The figure shows three views and two pictorial views of one solid part (mm, origin at its lowest corner). Answer the questions. Round coordinates to 2 decimals unless told otherwise and drop trailing zeros. Order: outer loops, then holes, each group sorted by start corner. A loop starts at its lowest first (then second) coordinate and runs counter-clockwise, first axis right, second up. Notation, with made-up numbers: (31, 88) - (77, 88) arc R13 ccw to (77, 94) - close; hole circle Ø7 at (-37.75, -13.75). An arc over 180 degrees is marked (long way). Use CSV: the item, a comma, the result in double quotes.
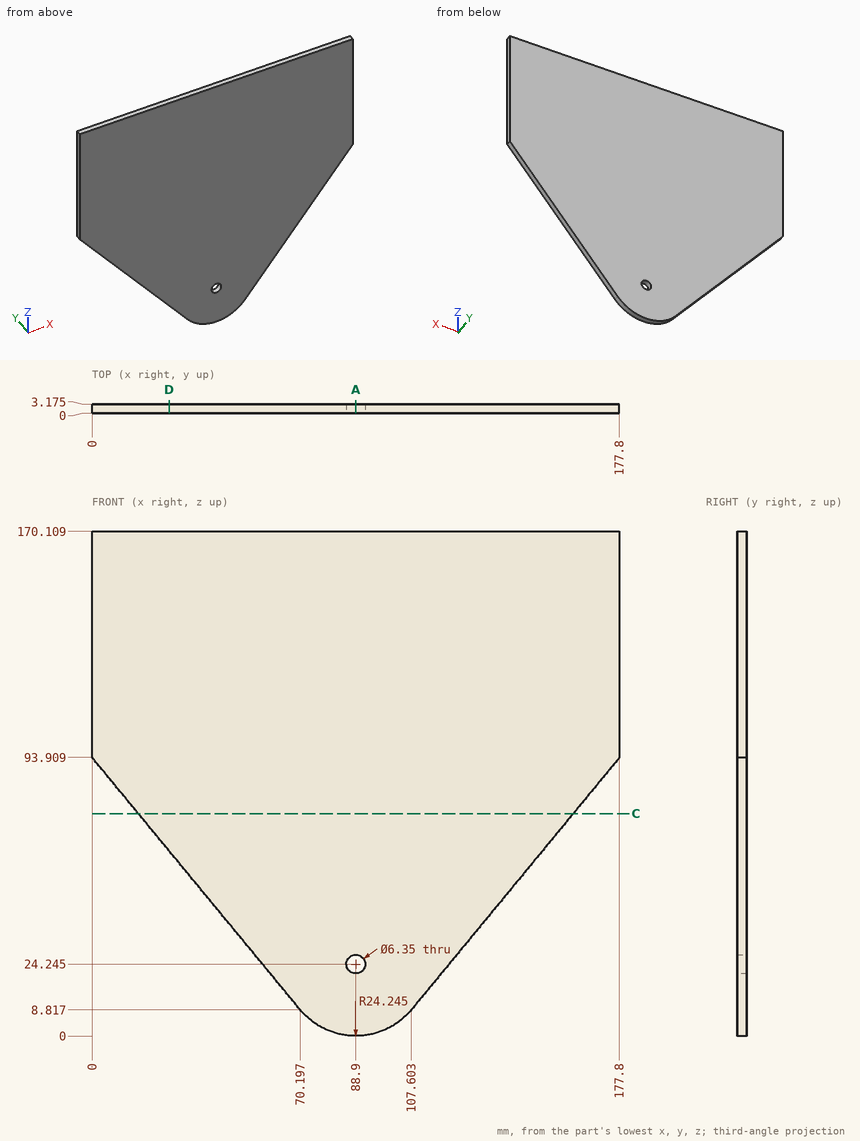
(1) Find the intervals of material crossed by L1, parallel to Z at x = 26, y = 2.2 (1 decimal); L2, parallel to X at y = 0.9, z = 19 (1 decimal); L3, parallel to Z at x = 135, y = 1.45 (1 decimal), in increasing order. Write a range as from..to.
Findings below:
L1,"z = 62.4..170.1"
L2,"x = 61.8..116"
L3,"z = 42..170.1"
(2) Find section D-D (x = 26). Determine the outline of the cut face in (y, z) (1 decimal).
Findings below:
outline,"(0, 62.4) - (3.2, 62.4) - (3.2, 170.1) - (0, 170.1) - close"
(3) Find section A-A (x = 88.9). Determine the outline of the cut face in (y, z) (1 decimal).
Findings below:
outline,"(0, 0) - (3.2, 0) - (3.2, 21.1) - (0, 21.1) - close; (0, 27.4) - (3.2, 27.4) - (3.2, 170.1) - (0, 170.1) - close"
(4) Each of these flat-tipped pins is pushed along its axis until it touches: pin 1 (5.5 mm diameter, centred on x = 88.9, z = 24.25, fed in from -Y); pin 2 (1 mm diameter, centred on y = 1, z = 35.5, fed in from +X); pin 3 (1 mm diameter, centred on x = 134, y = 2.5, fed in from -Z). Where does it stop, or does it pass through?
Findings below:
pin 1,"passes through"
pin 2,"stops at x = 130.03"
pin 3,"stops at z = 40.21"
(5) Find section C-C (z = 75). Determine the outline of the cut face in (x, y) (1 decimal).
Findings below:
outline,"(15.6, 0) - (162.2, 0) - (162.2, 3.2) - (15.6, 3.2) - close"
